```python
from build123d import *

# Parameters (mm, degrees)
CUT_EXTRUDE1_DEPTH = 2.38


with BuildPart() as part:
    # Sketch1 → Revolve1 (revolve)
    with BuildSketch(Plane.XY, mode=Mode.PRIVATE) as revolve1_sk:
        Polygon((0, 0), (30, 0), (30, 3), (4, 3), (4, 5), (0, 5), align=None)
    revolve(revolve1_sk.sketch.rotate(Axis((0, 0, 0), (1, 0, 0)), 90), axis=Axis((0, 0, 0), (1, 0, 0)))

    # Sketch2 → Cut-Extrude1 (cut)
    with BuildSketch(Plane.ZY):
        Polygon((2.886751346, 0), (1.443375673, 2.5), (-1.443375673, 2.5), (-2.886751346, 0), (-1.443375673, -2.5), (1.443375673, -2.5), align=None)
    extrude(amount=-CUT_EXTRUDE1_DEPTH, mode=Mode.SUBTRACT)


solid = part.part
```
Can you work these out from the model? Positions are in its coordinate system, mm. A direction names the side the tool comes from. Coordinates: 2 decimals unless noted, no trailing zeros. Loops run counter-clockwise (first coordinate to the right, second up) from the corner with the lowest first, then second, coordinate; pieces in that order, holes last. Notation, with made-up numbers: (21, 65) -> (65, 65) arc R31 cw to (65, 95) -> close; hole circle Ø8 at (69, -27). An arc over 180 degrees is marked (long way). Put each result on its own line as item: value. Start each with the question number.
Q1. I want a section at A-A (x = 2). Write out the boundary of the cut face in (y, z), plus the area to 3 significant figures.
Q2. I want a section at C-C (y = 4). Write out the boundary of the cut face in (x, z), plus the area to 3 significant figures.
Q3. Thinking about a two-plate mould opening in Y: for faces 4 (the face through (4, 3.3, 0.1)), 5 (the face through (2, 0, -5)), 6 (the face through (1, 2.5, 0)), 7 (the face through (1.173, -1.267, 2.155)), which applies, pulls with the +Y half, pulls with the -Y half, needs draft (parallel to the pull), parting line crosses it, or undercut?
Q4. I'm going to push flat-ended pins straight in: P1, Ø6, axis at x = 12, z = -2, coming from the -Y side; P2, Ø3, axis at x = 14, y = -0.5, coming from the +Z side; P3, Ø5, axis at x = 16, z = 3.5, coming from the -Y side. Where does each tip first touch, or does it pass through?
Q5. I want a section at B-B (z = 0). Write out the boundary of the cut face in (x, y), plus the area to 3 significant figures.
Q6. If I drill on line 1 (X direction, y = 2.25, z = 1.5); line 2 (X direction, y = -2.5, z = -2.75); line 3 (Y direction, x = 14, z = 2.5), over which ranges is the centre line in solid material (lowest first)? Write a range as [from, to].
Q7. I want a section at D-D (x = 13). Write out the boundary of the cut face in (y, z), plus the area to 3 significant figures.
Q8. For faces 1 (the face through (0, 2, 2)), 2 (the face through (16.82, -0.9, 2.86)), 3 (the face through (1, -2.5, 0)), which set-ups out of +Z, -Z, +X, -X, +Y, -Y let a thin tool reach every point of the face, with its end or its side?
Taken from the geometry:
1. outline: circle Ø10 at (0, 0); hole (-2.5, -1.44) -> (0, -2.89) -> (2.5, -1.44) -> (2.5, 1.44) -> (0, 2.89) -> (-2.5, 1.44) -> close
1. area: 56.9 mm2
2. outline: (0, -3) -> (4, -3) -> (4, 3) -> (0, 3) -> close
2. area: 24.0 mm2
3. face 4: needs draft
3. face 5: parting line crosses it
3. face 6: undercut
3. face 7: undercut
4. P1: stops at y = -3
4. P2: stops at z = 3
4. P3: stops at y = -2.83
5. outline: (0, -5) -> (4, -5) -> (4, -3) -> (30, -3) -> (30, 3) -> (4, 3) -> (4, 5) -> (0, 5) -> (0, 2.5) -> (2.38, 2.5) -> (2.38, -2.5) -> (0, -2.5) -> close
5. area: 184 mm2
6. line 1: x = [2.38, 30]
6. line 2: x = [0, 4]
6. line 3: y = [-1.66, 1.66]
7. outline: circle Ø6 at (0, 0)
7. area: 28.3 mm2
8. face 1: +Z, -Z, -X, +Y, -Y
8. face 2: +X
8. face 3: -X
